The listing builds one solid part. Answer for the finished solid, in the listing's coordinates (mm). A direction names the side the tool comes from. Give positions to 0.01 mm unless a question says otherwise; leave off trailing zeros. Write each loop counter-clockwise with the first axis right and the second up, starting at its lowest first coordinate (ties: lowest second). Pieces come first, ordered by that corner, then holes.
```python
from build123d import *

# Parameters (mm, degrees)
ESQUISSE6_R        = 25
ESQUISSE6_R_2      = 24
ESQUISSE8_R        = 26.000000000000007
ESQUISSE8_R_2      = 24.000000000000007
EXTRU_MINCE1_DEPTH = 1
EXTRU_MINCE2_START = 30
ESQUISSE9_R        = 26
ESQUISSE9_R_2      = 25
EXTRU_MINCE2_DEPTH = 30
CONG_1_R           = 1
CONG_2_R           = 1


with BuildPart() as part:
    # Balayage-Mince2: sweep along a path in Esquisse7
    with BuildLine(Plane(origin=(0, 0, 0), x_dir=(0, 0, -1), z_dir=(1, 0, 0))) as balayage_mince2_path:
        Line((0, 0), (-41.38142332276701, -3.47e-15))
        ThreePointArc((-41.38142332276701, -3.47e-15), (-62.08896052980016, 8.292906624346546), (-71.34811957162613, 28.58680647871081))
        Line((-71.34811957162613, 28.58680647871081), (-71.83715157767594, 38.95670512351683))
    # Esquisse6 → Balayage-Mince2 (sweep)
    with BuildSketch(Plane.XY):
        Circle(ESQUISSE6_R)
        Circle(ESQUISSE6_R_2, mode=Mode.SUBTRACT)
    sweep(path=balayage_mince2_path.line)



with BuildPart() as body_2:
    # Esquisse8 → Extru.-Mince1 (new body)
    with BuildSketch(Plane(origin=(0, 42.25049608966464, 1.9924828165681323), x_dir=(1, 0, 0), z_dir=(0, 0.9988898749619701, 0.047106450709639855))):
        with Locations((0, -69.92229124733788)):
            Circle(ESQUISSE8_R)
        with Locations((0, -69.92229124733788)):
            Circle(ESQUISSE8_R_2, mode=Mode.SUBTRACT)
    extrude(amount=EXTRU_MINCE1_DEPTH)


with BuildPart() as part_1:
    add(part.part)

    add(body_2.part)  # Extru.-Mince2 merges body 2
    # Esquisse9 → Extru.-Mince2 (add)
    with BuildSketch(Plane(origin=(0, 43.249385964626626, 2.039589267277776), x_dir=(1, 0, 0), z_dir=(0, 0.9988898749619701, 0.04710645070963987)).offset(EXTRU_MINCE2_START)):
        with Locations((0, -69.92229124733788)):
            Circle(ESQUISSE9_R)
        with Locations((0, -69.92229124733788)):
            Circle(ESQUISSE9_R_2, mode=Mode.SUBTRACT)
    extrude(amount=-EXTRU_MINCE2_DEPTH)

    # Congé1
    cong_1_edges = [part_1.edges().sort_by_distance(p)[0] for p in [
        (-25, 38.95670512351683, 71.8371515776759),
    ]]
    fillet(cong_1_edges, radius=CONG_1_R - 0.0001)  # a hair under: the kernel refuses the full size

    # Congé2
    cong_2_edges = [part_1.edges().sort_by_distance(p)[0] for p in [
        (-26.000000000000007, 38.956705123516834, 71.83715157767593),
    ]]
    fillet(cong_2_edges, radius=CONG_2_R)


solid = part_1.part
```
Item 1: Consider probe 1 along Y at (x, z) = (-0.5, 11) (3 decimals); probe 2 along Z at (x, y) = (-7, 65.5); probe 3 along Z at (x, y) = (3, 66.5). Determine where each line is inside the solid, lowest interval first.
Conclusion:
probe 1: y = -24.995 to -23.995, 23.995 to 24.995
probe 2: z = 48.02 to 49.06, 97.12 to 98.16
probe 3: z = 47.28 to 48.29, 97.98 to 98.99
Item 2: Which of the six approach directions +Z, -Z, +X, -X, +Y, -Y give full straight-line access (tool end or side, diameter ignored) to faces 4 (the face through (-22.3, 40.4, 62.5)), 5 (the face through (-23.977, 1.055, 20.98)), 6 (the face through (-9.4, 22.3, 0))?
Conclusion:
face 4: none
face 5: -Z
face 6: -Z, +X, -X, +Y, -Y
Item 3: Each of these flat-tipped pins is pushed along its axis until it touches: P1, Ø12, axis at x = -17.5, y = -9, coming from the -Z side; P2, Ø6, axis at x = -4, z = 48, coming from the -Y side; P3, Ø12, axis at x = 5.5, y = 12.5, coming from the +Z side; P4, Ø8, axis at x = -2.5, z = 82.5, coming from the +Y side. Where does it stop, or does it pass through?
Conclusion:
P1: stops at z = 0
P2: stops at y = -24.75
P3: stops at z = 94.86
P4: stops at y = 0.63
Item 4: A cutting plane is placed at A-A, the plane z = 34. Give the vertices of the cut face in (x, y), plus the area to 3 significant figures.
Conclusion:
outline: circle Ø50 at (0, 0); hole circle Ø48 at (0, 0)
area: 154 mm2
Item 5: Determine the mould class of faces 1 (the face through (23.846, 55.502, 65.1)), 2 (the face through (-13.603, 70.926, 52.015)), 3 (the face through (23.846, 7.509, 20.98)) for opening direction Y: pulls with the +Y half, pulls with the -Y half, needs draft (parallel to the pull), parting line crosses it, or undercut.
Conclusion:
face 1: undercut
face 2: pulls with the +Y half
face 3: parting line crosses it
